Job drawing, mm, ordinate dimensions from the low corner. One solid piece. A direction names the side the tool comes from. Round coordinates to 2 decimals unless told otherwise and drop trailing zeros. Order: outer loops, then holes, each group sorted by start corner. A loop starts at its lowest first (then second) coordinate and runs counter-clockwise, first axis right, second up. Notation, with made-up numbers: (72, 5) -> (114, 5) arc R21 cw to (114, 34) -> close; hole circle Ø10 at (-5.5, -30.5). An arc over 180 degrees is marked (long way). Use CSV: the item, a comma, the result in double quotes.
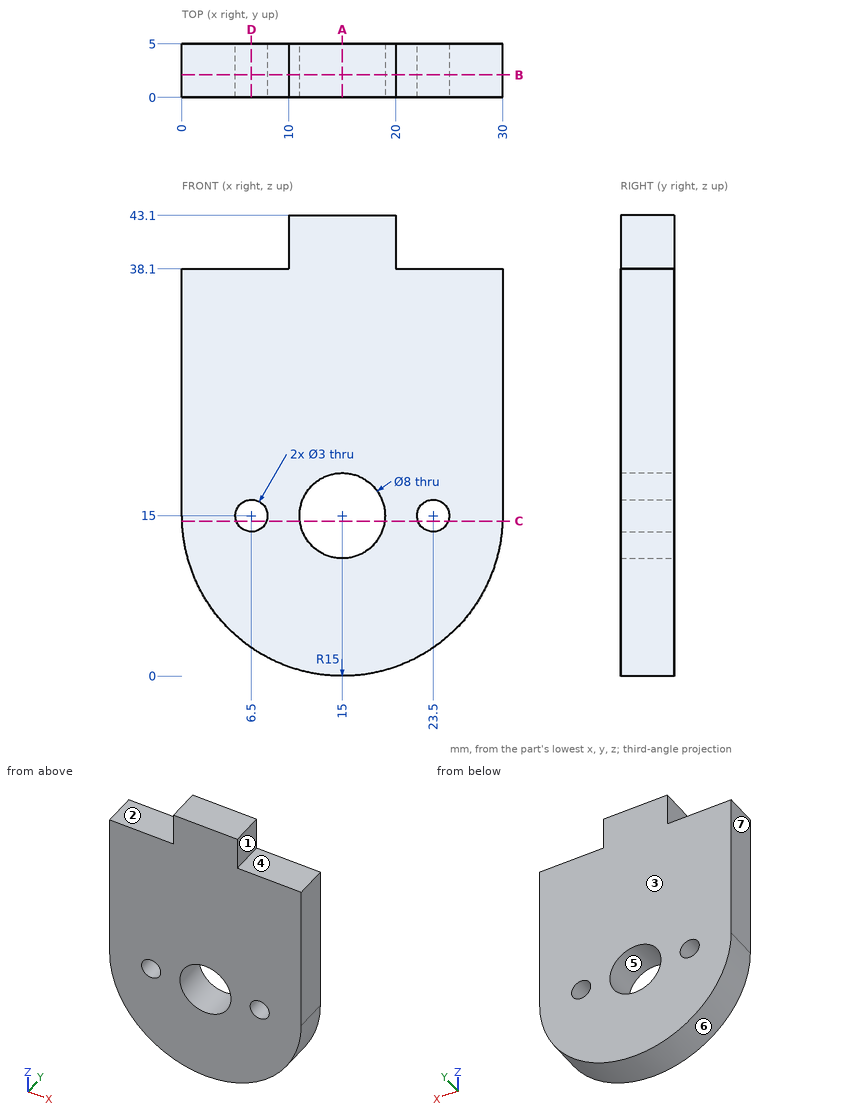
(1) Which spindle directions (+Z, -Z, +X, -X, +Y, -Y) get a long thin tool onto all of the face, cutting with end or side? Do the marked faces 1, 2 and 3. Say none if no direction does.
Reply:
face 1,"+Z, +X, +Y, -Y"
face 2,"+Z, -X, +Y, -Y"
face 3,"+Z, -Z, +X, -X, +Y"
(2) Cut at D-D, the plane x = 6.5. Give the cut face in (y, z), then the cut area to 3 significant figures.
Reply:
outline,"(0, 2.64) -> (5, 2.64) -> (5, 13.5) -> (0, 13.5) -> close; (0, 16.5) -> (5, 16.5) -> (5, 38.1) -> (0, 38.1) -> close"
area,"162 mm2"
(3) Probe probe 1 along X at (y, z) = (2.4, 15); probe 2 along Z at (x, y) = (15, 3.9); probe 3 along X at (y, z) = (0.85, 13). List the from-to ranges inside material, lowest first. Write a range as [from, to].
Reply:
probe 1,"[0, 5], [8, 11], [19, 22], [25, 30]"
probe 2,"[0, 11], [19, 43.1]"
probe 3,"[0.13, 11.54], [18.46, 29.87]"
(4) Cut at A-A, the plane x = 15. Give the cut face in (y, z).
Reply:
outline,"(0, 0) -> (5, 0) -> (5, 11) -> (0, 11) -> close; (0, 19) -> (5, 19) -> (5, 43.1) -> (0, 43.1) -> close"
(5) Cut at B-B, the plane y = 2.1. Give the cut face in (x, z).
Reply:
outline,"(0, 15) arc R15 ccw to (30, 15) -> (30, 38.1) -> (20, 38.1) -> (20, 43.1) -> (10, 43.1) -> (10, 38.1) -> (0, 38.1) -> close; hole circle Ø3 at (6.5, 15); hole circle Ø8 at (15, 15); hole circle Ø3 at (23.5, 15)"
(6) Pull direction X, two halves, no side cores. Call the marked faces 4, 5, 6 and 7: released by +X, released by -X, zero draft, split by the parting line, or undercut.
Reply:
face 4,"zero draft"
face 5,"undercut"
face 6,"split by the parting line"
face 7,"released by -X"
(7) Drop flat-ended pins along their axis: P1, Ø6.5, axis at x = 15, z = 15, coming from the -Y side; P2, Ø1.5, axis at y = 1.5, z = 40, coming from the +X side; P3, Ø2, axis at x = 7, y = 1, coming from the +Z side. Give the stop position or say it passes through.
Reply:
P1,"through"
P2,"x = 20"
P3,"z = 38.1"
(8) Cut at C-C, the plane z = 14.5. Give the cut face in (x, y).
Reply:
outline,"(0.01, 0) -> (5.09, 0) -> (5.09, 5) -> (0.01, 5) -> close; (7.91, 0) -> (11.03, 0) -> (11.03, 5) -> (7.91, 5) -> close; (18.97, 0) -> (22.09, 0) -> (22.09, 5) -> (18.97, 5) -> close; (24.91, 0) -> (29.99, 0) -> (29.99, 5) -> (24.91, 5) -> close"
